Work out the finished part from the listing and answer in its coordinate system (mm). Face numbers are marked on the shaded views. A direction names the side the tool comes from. Give positions to 0.01 mm unless a question says otherwise; leave off trailing zeros. Order: outer loops, then holes, each group sorted by start corner. A loop starts at its lowest first (then second) coordinate and runs counter-clockwise, first axis right, second up. Notation, with made-up numbers: (68, 54) - (82, 54) arc R33 cw to (82, 86) - close; hole circle Ø3 at (27.5, 14). An arc over 180 degrees is marked (long way). Put each result on its own line as item: value.
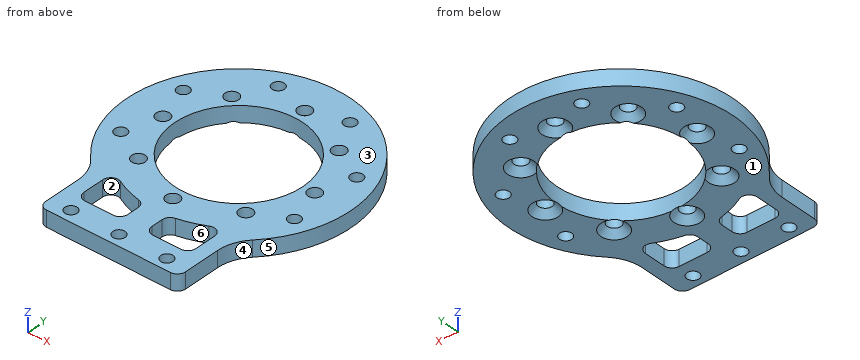
```python
from build123d import *

# Parameters (mm, degrees)
SKETCH_2_R                   = 28
SKETCH_2_R_2                 = 1.525
SKETCH_2_W                   = 35
SKETCH_2_H                   = 15.642507006
EXTRUDE_1_DEPTH              = 4
SKETCH_3_R                   = 16
CUT_EXTRUDE_1_DEPTH          = 47.97073557
SKETCH_4_R                   = 1.525
CUT_EXTRUDE_2_DEPTH          = 47.97073557
FILLET_1_R                   = 2
FILLET_2_R                   = 10
CUT_EXTRUDE_START            = -4
CUT_EXTRUDE_3_DEPTH          = 4
FILLET_3_R                   = 2
SKETCH_7_R                   = 1.525
CUT_EXTRUDE_4_DEPTH          = 47.97073557
HOLE_WIZARD_M3_1_D           = 3.4
HOLE_WIZARD_M3_1_CSINK_D     = 6.6
HOLE_WIZARD_M3_1_CSINK_ANGLE = 90


# Read off the part's stored shape, not the designer's step: 切除-拉伸3
with BuildPart() as part:
    # 草图2 → 凸台-拉伸1 (new body)
    # profile 1 of 2: a face of its own
    with BuildSketch(Plane.XY):
        Circle(SKETCH_2_R)
        with Locations((19, 0)):
            Circle(SKETCH_2_R_2, mode=Mode.SUBTRACT)
        with Locations((13.435028843, -13.435028843)):
            Circle(SKETCH_2_R_2, mode=Mode.SUBTRACT)
        with Locations((0, -19)):
            Circle(SKETCH_2_R_2, mode=Mode.SUBTRACT)
        with Locations((-13.435028843, -13.435028843)):
            Circle(SKETCH_2_R_2, mode=Mode.SUBTRACT)
        with Locations((-19, 0)):
            Circle(SKETCH_2_R_2, mode=Mode.SUBTRACT)
        with Locations((-13.435028843, 13.435028843)):
            Circle(SKETCH_2_R_2, mode=Mode.SUBTRACT)
        with Locations((0, 19)):
            Circle(SKETCH_2_R_2, mode=Mode.SUBTRACT)
        with Locations((13.435028843, 13.435028843)):
            Circle(SKETCH_2_R_2, mode=Mode.SUBTRACT)
    # profile 2 of 2: a face of its own
    with BuildSketch(Plane.XY):
        with Locations((0, -29.678746497)):
            Rectangle(SKETCH_2_W, SKETCH_2_H)
    extrude(amount=EXTRUDE_1_DEPTH)

    # 草图3 → 切除-拉伸1 (cut, through all)
    with BuildSketch(Plane.XY.offset(4)):
        Circle(SKETCH_3_R)
    extrude(amount=-CUT_EXTRUDE_1_DEPTH, mode=Mode.SUBTRACT)

    # 草图4 → 切除-拉伸2 (cut, through all)
    with BuildSketch(Plane.XY.offset(4)):
        with Locations((0, -34.5)):
            Circle(SKETCH_4_R)
        with Locations((-12, -34.5)):
            Circle(SKETCH_4_R)
        with Locations(Location((12, -34.5, 0), (0, 0, 180))):
            Circle(SKETCH_4_R)
    extrude(amount=-CUT_EXTRUDE_2_DEPTH, mode=Mode.SUBTRACT)

    # 圆角1
    fillet_1_edges = [part.edges().sort_by_distance(p)[0] for p in [
        (17.5, -37.5, 2),
        (-17.5, -37.5, 2),
    ]]
    fillet(fillet_1_edges, radius=FILLET_1_R)

    # 圆角2
    fillet_2_edges = [part.edges().sort_by_distance(p)[0] for p in [
        (17.5, -21.857492994, 2),
        (-17.5, -21.857492994, 2),
    ]]
    fillet(fillet_2_edges, radius=FILLET_2_R)

    # 切除-拉伸3 outline → 切除-拉伸3 (cut)
    with BuildSketch(Plane.XY.offset(4).offset(CUT_EXTRUDE_START)):
        with BuildLine():
            ThreePointArc((14, -19.49358869), (8.769929005, -22.340285254), (3, -23.8117618))
            Line((3, -23.8117618), (3, -30.49358869))
            Line((3, -30.49358869), (14, -30.49358869))
            Line((14, -30.49358869), (14, -19.49358869))
        make_face()
        with BuildLine():
            ThreePointArc((-3, -23.8117618), (-8.769929005, -22.340285254), (-14, -19.49358869))
            Line((-14, -19.49358869), (-14, -30.49358869))
            Line((-14, -30.49358869), (-3, -30.49358869))
            Line((-3, -30.49358869), (-3, -23.8117618))
        make_face()
    extrude(amount=CUT_EXTRUDE_3_DEPTH, mode=Mode.SUBTRACT)

    # 圆角3
    fillet_3_edges = [part.edges().sort_by_distance(p)[0] for p in [
        (-14, -19.49358869, 2),
        (-3, -23.8117618, 2),
        (-3, -30.49358869, 2),
        (-14, -30.49358869, 2),
        (3, -23.8117618, 2),
        (14, -19.49358869, 2),
        (14, -30.49358869, 2),
        (3, -30.49358869, 2),
    ]]
    fillet(fillet_3_edges, radius=FILLET_3_R)

    # 草图7 → 切除-拉伸4 (cut, through all)
    with BuildSketch(Plane.XY.offset(4)):
        with Locations((21.711169014, 8.993060661)):
            Circle(SKETCH_7_R)
        with Locations((21.711169014, -8.993060661)):
            Circle(SKETCH_7_R)
        with Locations((-21.711169014, -8.993060661)):
            Circle(SKETCH_7_R)
        with Locations((-21.711169014, 8.993060661)):
            Circle(SKETCH_7_R)
        with Locations((-8.993060661, 21.711169014)):
            Circle(SKETCH_7_R)
        with Locations((8.993060661, 21.711169014)):
            Circle(SKETCH_7_R)
    extrude(amount=-CUT_EXTRUDE_4_DEPTH, mode=Mode.SUBTRACT)

    # M3 开槽沉头木螺钉的锥形沉头孔1 (through all)
    with Locations(Plane(origin=(0, 0, 0), x_dir=(-1, 0, 0), z_dir=(0, 0, -1))):
        with Locations((-19, 0), (-13.435028842, 13.435028843), (0, 19), (13.435028843, 13.435028843), (19, 0), (13.435028843, -13.435028843), (0, -19), (-13.435028843, -13.435028843)):
            CounterSinkHole(HOLE_WIZARD_M3_1_D / 2, HOLE_WIZARD_M3_1_CSINK_D / 2, counter_sink_angle=HOLE_WIZARD_M3_1_CSINK_ANGLE)


solid = part.part
```
(1) Given pin 1 (4 mm diameter, centred on x = -13.44, y = -13.44, fed in from -Z); pin 2 (4.5 mm diameter, centred on x = 19, y = 0, fed in from -Z); pin 3 (2 mm diameter, centred on y = -31.5, z = 1.5, fed in from -X), each flat-ended and moving along its own axis, determine where each tip first touches the part or whether it passes through.
Geometry check:
pin 1: stops at z = 1.29
pin 2: stops at z = 1.05
pin 3: stops at x = -17.5
(2) A tool of negligible diameter and unlimited length cuts with its end or side. For the marked faces 1 and 2, from which of +Z, -Z, +X, -X, +Y, -Y can it reach the whole face along a straight path? Write none if from no direction.
Geometry check:
face 1: -Z, +X, -X, +Y, -Y
face 2: +Z, -Z
(3) Section C-C, the plane y = 19 is taken. Write down the section's boundary in (x, z), then the cut area to 3 significant figures.
Geometry check:
outline: (-20.57, 0) - (-3.3, 0) - (-1.7, 1.6) - (-1.7, 4) - (-20.57, 4) - close; (1.7, 1.6) - (3.3, 0) - (20.57, 0) - (20.57, 4) - (1.7, 4) - close
area: 148 mm²
(4) Straight lines are drawn through the part: line 1 (X direction, y = -28, z = 1.45); line 2 (Y direction, x = 0, z = 2.75) (3 decimals); line 3 (X direction, y = -12, z = 2.5). For each, find the intervals that lie inside material, in ascending order.
Geometry check:
line 1: x = -17.5 to -14, -3 to 3, 14 to 17.5
line 2: y = -37.5 to -36.025, -32.975 to -20.7, -17.3 to -16, 16 to 17.3, 20.7 to 28
line 3: x = -25.3 to -14.35, -12.52 to -10.58, 10.58 to 12.52, 14.35 to 25.3
(5) Determine the mould class of the marked faces 3, 4, 5 and 6 for opening direction Y: pulls with the +Y half, pulls with the -Y half, needs draft (parallel to the pull), parting line crosses it, or undercut.
Geometry check:
face 3: needs draft
face 4: pulls with the -Y half
face 5: parting line crosses it
face 6: undercut
(6) Section B-B, the plane y = 0 is taken. Write down the section's boundary in (x, z).
Geometry check:
outline: (-28, 0) - (-22.3, 0) - (-20.7, 1.6) - (-20.7, 4) - (-28, 4) - close; (-17.3, 1.6) - (-16, 0.3) - (-16, 4) - (-17.3, 4) - close; (16, 0.3) - (17.3, 1.6) - (17.3, 4) - (16, 4) - close; (20.7, 1.6) - (22.3, 0) - (28, 0) - (28, 4) - (20.7, 4) - close
(7) Section A-A, the plane x = 0 is taken. Write down the section's boundary in (y, z) (3 decimals), then the cut area to 3 significant figures.
Geometry check:
outline: (-37.5, 0) - (-36.025, 0) - (-36.025, 4) - (-37.5, 4) - close; (-32.975, 0) - (-22.3, 0) - (-20.7, 1.6) - (-20.7, 4) - (-32.975, 4) - close; (-17.3, 1.6) - (-16, 0.3) - (-16, 4) - (-17.3, 4) - close; (16, 0.3) - (17.3, 1.6) - (17.3, 4) - (16, 4) - close; (20.7, 1.6) - (22.3, 0) - (28, 0) - (28, 4) - (20.7, 4) - close
area: 89.6 mm²
(8) Section D-D, the plane x = 19 is taken. Write down the section's boundary in (y, z).
Geometry check:
outline: (-20.96, 0) - (-3.3, 0) - (-1.7, 1.6) - (-1.7, 4) - (-20.96, 4) - close; (1.7, 1.6) - (3.3, 0) - (20.57, 0) - (20.57, 4) - (1.7, 4) - close
